from build123d import *
from OCP.BRepFilletAPI import BRepFilletAPI_MakeChamfer

# Parameters (mm, degrees)
DOWELSUPPORT_DEPTH       = 1.905
DOWELSUPPORT_DEPTH_BACK  = 1.27
SKETCH3_R                = 3.81
SKETCH5_W                = 9.525
SKETCH5_H                = 19.05
SLIDERDOWELSUPPORT_DEPTH = 1.27
STRINGDOWELSUPPORT_DEPTH = 1.27
SKETCH9_W                = 6.35
SKETCH9_H                = 3
TABSUPPORT_DEPTH         = 1.27
INTERSUPPORT_DEPTH       = 1.27
DOWELHOLES_DEPTH         = 25.48367648
DOWELHOLES_DEPTH_BACK    = 25.48367648
SKETCH11_R               = 1.600000102
BOSS_EXTRUDE1_START      = -1.27
SKETCH11_2_R             = 1.600000102
BOSS_EXTRUDE1_DEPTH      = 0.254
SKETCH14_W               = 6.35
SKETCH14_H               = 3
TABBASE_DEPTH            = 1.27
SKETCH15_W               = 6.35
SKETCH15_H               = 3
TABDRAFT_DEPTH           = 1.73
TABDRAFT_DRAFT           = 5
TABDRAFT_PROFILE_2_DEPTH = 1.73
TABDRAFT_PROFILE_2_DRAFT = 5
CHAMFER1_SIZE            = 2.54
CUT_EXTRUDE2_DEPTH       = 3
CHAMFER2_SIZE            = 0.508
CHAMFER2_SIZE2           = 1.016


with BuildPart() as part:
    # Sketch3 → DowelSupport (new, two sides: drawn at the far end of the back side and taken through both)
    with BuildSketch(Plane(origin=(0, 0, 0), x_dir=(0, 0, -1), z_dir=(1, 0, 0)).offset(-DOWELSUPPORT_DEPTH_BACK)):
        with Locations((-3.175, 14.53375)):
            Circle(SKETCH3_R)
    extrude(amount=DOWELSUPPORT_DEPTH + DOWELSUPPORT_DEPTH_BACK)



with BuildPart() as body_2:
    # Sketch5 → SliderDowelSupport (new, symmetric)
    with BuildSketch(Plane(origin=(0, 0, 0), x_dir=(0, 0, -1), z_dir=(1, 0, 0))):
        with Locations((-1.5875, 0)):
            Rectangle(SKETCH5_W, SKETCH5_H)
    extrude(amount=SLIDERDOWELSUPPORT_DEPTH, both=True)


with BuildPart() as body_3:
    # Sketch8 → StringDowelSupport (new, symmetric)
    with BuildSketch(Plane(origin=(0, 0, 0), x_dir=(0, 0, -1), z_dir=(1, 0, 0))):
        with BuildLine():
            Line((4.6355, 18.542), (8.0645, 18.542))
            ThreePointArc((8.0645, 18.542), (10.6045, 16.002), (8.0645, 13.462))
            Line((8.0645, 13.462), (4.6355, 13.462))
            ThreePointArc((4.6355, 13.462), (2.0955, 16.002), (4.6355, 18.542))
        make_face()
    extrude(amount=STRINGDOWELSUPPORT_DEPTH, both=True)


with BuildPart() as part_1:
    add(part.part)

    add(body_3.part)  # TabSupport merges body 3
    # Sketch9 → TabSupport (add, symmetric)
    with BuildSketch(Plane(origin=(0, 0, 0), x_dir=(0, 0, -1), z_dir=(1, 0, 0))):
        with Locations((0, 15.24)):
            Rectangle(SKETCH9_W, SKETCH9_H)
        with Locations((12.7, 15.24)):
            Rectangle(SKETCH9_W, SKETCH9_H)
    extrude(amount=TABSUPPORT_DEPTH, both=True)


    add(body_2.part)  # InterSupport merges body 2
    # Sketch10 → InterSupport (add, symmetric)
    with BuildSketch(Plane(origin=(0, 0, 0), x_dir=(0, 0, -1), z_dir=(1, 0, 0))):
        Polygon((-6.35, 9.525), (-5.696013987, 14.843731414), (-3.644260291, 17.030026182), (4.166239709, 18.498276182), (8.657140431, 18.471894192), (15.875, 16.74), (15.875, 13.74), (3.175, 3.175), (3.175, 9.525), align=None)
    extrude(amount=INTERSUPPORT_DEPTH, both=True)

    # Sketch11 → DowelHoles (cut, two sides: drawn at the far end of the back side and taken through both)
    with BuildSketch(Plane(origin=(0, 0, 0), x_dir=(0, 0, -1), z_dir=(1, 0, 0)).offset(-DOWELHOLES_DEPTH_BACK)):
        with Locations((-3.175, 14.53375)):
            Circle(SKETCH11_R)
        with BuildLine():
            Line((6.04239599, 15.24), (6.65760401, 15.24))
            ThreePointArc((6.65760401, 15.24), (9.664500102, 16.002), (6.65760401, 16.764))
            Line((6.65760401, 16.764), (6.04239599, 16.764))
            ThreePointArc((6.04239599, 16.764), (3.035499898, 16.002), (6.04239599, 15.24))
        make_face()
    extrude(amount=DOWELHOLES_DEPTH + DOWELHOLES_DEPTH_BACK, mode=Mode.SUBTRACT)

    # Sketch11<2> → Boss-Extrude1 (add)
    with BuildSketch(Plane(origin=(0, 0, 0), x_dir=(0, 0, -1), z_dir=(1, 0, 0)).offset(BOSS_EXTRUDE1_START)):
        with BuildLine():
            Line((6.04239599, 15.24), (6.65760401, 15.24))
            ThreePointArc((6.65760401, 15.24), (9.664500102, 16.002), (6.65760401, 16.764))
            Line((6.65760401, 16.764), (6.04239599, 16.764))
            ThreePointArc((6.04239599, 16.764), (3.035499898, 16.002), (6.04239599, 15.24))
        make_face()
        with Locations((-3.175, 14.53375)):
            Circle(SKETCH11_2_R)
    extrude(amount=BOSS_EXTRUDE1_DEPTH)

    # Sketch14 → TabBase (add)
    with BuildSketch(Plane.ZY.offset(1.27)):
        with Locations((-12.7, 15.24)):
            Rectangle(SKETCH14_W, SKETCH14_H)
        with Locations((0, 15.24)):
            Rectangle(SKETCH14_W, SKETCH14_H)
    extrude(amount=TABBASE_DEPTH)


with BuildPart() as tabdraft_tool:
    # Sketch15 → TabDraft (with draft: the straight prism first)
    with BuildSketch(Plane.ZY.offset(2.54)):
        with Locations((0, 15.24)):
            Rectangle(SKETCH15_W, SKETCH15_H)
    extrude(amount=TABDRAFT_DEPTH)
    # TabDraft: the draft: its side faces are tilted about the plane it starts from
    tabdraft_sides = [tabdraft_tool.faces().sort_by_distance(p)[0] for p in [
        (-3.405, 15.24, -3.175),
        (-3.405, 13.74, 0),
        (-3.405, 15.24, 3.175),
        (-3.405, 16.74, 0),
    ]]
    draft(tabdraft_sides, Plane.ZY.offset(2.54), TABDRAFT_DRAFT)


with BuildPart() as part_2:
    add(part_1.part)

    # TabDraft: add tabdraft_tool
    add(tabdraft_tool.part)


with BuildPart() as tabdraft_profile_2_tool:
    # Sketch15 → TabDraft profile 2 (with draft: the straight prism first)
    with BuildSketch(Plane.ZY.offset(2.54)):
        with Locations((-12.7, 15.24)):
            Rectangle(SKETCH15_W, SKETCH15_H)
    extrude(amount=TABDRAFT_PROFILE_2_DEPTH)
    # TabDraft profile 2: the draft: its side faces are tilted about the plane it starts from
    tabdraft_profile_2_sides = [tabdraft_profile_2_tool.faces().sort_by_distance(p)[0] for p in [
        (-3.405, 15.24, -15.875),
        (-3.405, 13.74, -12.7),
        (-3.405, 15.24, -9.525),
        (-3.405, 16.74, -12.7),
    ]]
    draft(tabdraft_profile_2_sides, Plane.ZY.offset(2.54), TABDRAFT_PROFILE_2_DRAFT)


with BuildPart() as part_3:
    add(part_2.part)

    # TabDraft profile 2: add tabdraft_profile_2_tool
    add(tabdraft_profile_2_tool.part)

    # Chamfer1
    chamfer1_edges = [part_3.edges().sort_by_distance(p)[0] for p in [
        (1.27, 8.4575, -9.525),
    ]]
    chamfer(chamfer1_edges, length=CHAMFER1_SIZE - 0.0001)  # a hair under: the kernel refuses the full size

    # Mirror1: part across plane


with BuildPart() as part_4:
    add(part_3.part)
    add(part_3.part.mirror(Plane.ZX))

    # Sketch17 → Cut-Extrude2 (cut)
    with BuildSketch(Plane.XY.offset(6.35)):
        Polygon((-1.27, -4.006469684), (1.27, -2.54), (1.27, 2.54), (-1.27, 4.006469684), align=None)
    extrude(amount=-CUT_EXTRUDE2_DEPTH, mode=Mode.SUBTRACT)

    # Chamfer2: one chamfer whose edges measure the first distance from different faces: ONE call of the kernel's chamfer builder (chamfer() names one face for all edges)
    chamfer2_edges_1 = [part_4.edges().sort_by_distance(p)[0] for p in [
        (0, -3.273234842, 6.35),
    ]]
    chamfer2_side_1 = [part_4.faces().sort_by_distance(p)[0] for p in [
        (0.049650417, -6.38478458, 6.35),
    ]]
    chamfer2_edges_2 = [part_4.edges().sort_by_distance(p)[0] for p in [
        (0, 3.273234842, 6.35),
    ]]
    chamfer2_side_2 = [part_4.faces().sort_by_distance(p)[0] for p in [
        (0.049650417, 6.38478458, 6.35),
    ]]
    chamfer2 = BRepFilletAPI_MakeChamfer(part_4.part.solid().wrapped)
    for e in chamfer2_edges_1:
        chamfer2.Add(CHAMFER2_SIZE, CHAMFER2_SIZE2, e.wrapped, chamfer2_side_1[0].wrapped)  # the first distance lies on this face
    for e in chamfer2_edges_2:
        chamfer2.Add(CHAMFER2_SIZE, CHAMFER2_SIZE2, e.wrapped, chamfer2_side_2[0].wrapped)  # the first distance lies on this face
    add(Compound.cast(chamfer2.Shape()), mode=Mode.REPLACE)


solid = part_4.part
Geometry: final body of the model. Coordinates: model frame, mm. A direction names the side the tool comes from. Round coordinates to 2 decimals unless told otherwise and drop trailing zeros. Write each loop counter-clockwise with the first axis right and the second up, starting at its lowest first coordinate (ties: lowest second). Pieces come first, ordered by that corner, then holes. Notation, with made-up numbers: M 31,17 L 75,17 A34 cw 75,56 Z; hole C 49.5,-35 d6. An arc over 180 degrees is marked long. Write item = value, one per line.
Item 1: Pin query (flat end, axial travel): P1, Ø0.8, axis at x = 0, y = 7, coming from the +Z side; P2, Ø2.5, axis at y = -16, z = -7.5, coming from the +X side; P3, Ø3, axis at x = 1, y = -14, coming from the +Z side (3 decimals); P4, Ø1.6, axis at y = 14.5, z = 2.5, coming from the +X side. Return the tip coordinate at first contact, or that it passes through.
Findings:
P1 = 6.35
P2 = 1.27
P3 = 6.985
P4 = -1.02
Item 2: Access query for faces 1 (the face through (-2, 13.74, 0)), 2 (the face through (-2, -15, 3.175)), 3 (the face through (0, -6, 6.35)), 4 (the face through (-2, 15, -9.525)), 5 (the face through (-1.016, -16, -6)). Directions: +Z, -Z, +X, -X, +Y, -Y. A direction counts if a zero-diameter tool reaches every point of the face in a straight line with its end or side. Return the directions, or none.
Findings:
face_1 = +Z, -Z, -X
face_2 = +Z, -X, +Y, -Y
face_3 = +Z, +X, -X
face_4 = -X, +Y, -Y
face_5 = +X
Item 3: Section query C-C on y = -1. Return loops of the section in (x, z) (3 decimals), then the cut area to 3 significant figures.
Findings:
outline = M -1.27,-3.175 L 1.27,-3.175 L 1.27,3.35 L -1.27,3.35 Z
area = 16.6 mm^2
Item 4: Pull-direction query (Y, two-part tool) for faces 6 (the face through (0.02, 10.76, 6.2)), 7 (the face through (-3.4, 15.2, -3.1)), 8 (the face through (-3.393, -16.665, -0.044)); classes: pulls with the +Y half, pulls with the -Y half, needs draft (parallel to the pull), parting line crosses it, or undercut.
Findings:
face_6 = undercut
face_7 = needs draft
face_8 = pulls with the -Y half
Item 5: Section query A-A on x = -3.25. Return loops of the section in (y, z).
Findings:
outline = M -16.68,-15.81 L -13.8,-15.81 L -13.8,-9.59 L -16.68,-9.59 Z; M -16.68,-3.11 L -13.8,-3.11 L -13.8,3.11 L -16.68,3.11 Z; M 13.8,-15.81 L 16.68,-15.81 L 16.68,-9.59 L 13.8,-9.59 Z; M 13.8,-3.11 L 16.68,-3.11 L 16.68,3.11 L 13.8,3.11 Z
Item 6: Material intervals for line 1 along Y through (x, z) = (0.25, -4.5); line 2 along Z through (x, y) = (-0.25, -15); line 3 along Y through (x, z) = (-2.5, -10.5), sorted ascending. Write a range as [from, to].
Findings:
line_1 = [-18.54, -17.6], [-14.41, -6.25], [6.25, 14.41], [17.6, 18.54]
line_2 = [-15.79, -9.31], [-6.82, -5.88], [-3.39, 1.64], [4.71, 6.96]
line_3 = [-16.74, -13.74], [13.74, 16.74]
Item 7: Section query D-D on z = 0. Return loops of the section in (x, y) (3 decimals), then the cut area to 3 significant figures.
Findings:
outline = M -4.27,-16.589 L -2.54,-16.74 L -1.27,-16.74 L -1.27,-17.715 L 1.27,-17.715 L 1.27,-16.64 L 1.905,-16.64 L 1.905,-12.428 L 1.27,-12.428 L 1.27,12.428 L 1.905,12.428 L 1.905,16.64 L 1.27,16.64 L 1.27,17.715 L -1.27,17.715 L -1.27,16.74 L -2.54,16.74 L -4.27,16.589 L -4.27,13.891 L -2.54,13.74 L -1.27,13.74 L -1.27,-13.74 L -2.54,-13.74 L -4.27,-13.891 Z
area = 113 mm^2
